from build123d import *

# Parameters (mm, degrees)
F0_W     = 65
F0_H     = 110
F1_DEPTH = 1.6
F2_D     = 3.6


with BuildPart() as f1:
    # F0 (on Top) → F1 (new body)
    with BuildSketch(Plane.XY):
        with Locations((32.5, 55)):
            Rectangle(F0_W, F0_H)
    extrude(amount=F1_DEPTH)

    # F2 (through all)
    with Locations(Plane(origin=(0, 0, 0), x_dir=(1, 0, 0), z_dir=(0, 0, -1))):
        with Locations((3.81, -94.76), (61.19, -94.76), (3.81, -3.81), (61.19, -3.81)):
            Hole(F2_D / 2)


solid = f1.part
For this review, take the finished solid that the model builds, in its own axes (mm). Give positions to 0.01 mm unless a question says otherwise; leave off trailing zeros. Order: outer loops, then holes, each group sorted by start corner. A loop starts at its lowest first (then second) coordinate and runs counter-clockwise, first axis right, second up. Notation, with made-up numbers: M 7,-11 L 16,-11 A9 cw 16,-1 Z; hole C 60.5,-14.5 d2. An arc over 180 degrees is marked long. Answer in a Markdown table with one row per item. Add a question column.
(1) Consider section B-B on x = 61.19. State the section outline as (y, z) points.
(2) Wall thickness on probe 1 along X at (y, z) = (94.76, 0.8); probe 2 along Y at (x, z) = (61.19, 0.75): over which ranges is each line inside the solid? List them lowest first. Write a range as [from, to].
(3) Consider section A-A on y = 94.76. State the section outline as (x, z) points, and give its area (3 significant figures).
(4) Mouldability with a two-part tool opening along Y and no side actions: class faces 1 (the face through (60.359, 5.407, 0.811)), 2 (the face through (32, 56, 1.6)) as +Y half, -Y half, draft (parallel to the pull), parting line (faces both ways), or undercut.
(5) For pin 1 (4 mm diameter, centred on x = 61.19, y = 3.81, fed in from -Z); pin 2 (2 mm diameter, centred on x = 3.81, y = 3.81, fed in from +Z), all flat-tipped, find the tip position at first contact; note any pin that passes through.
Evaluation:
| question | item | result |
|---|---|---|
| 1 | outline | M 0,0 L 2.01,0 L 2.01,1.6 L 0,1.6 Z; M 5.61,0 L 92.96,0 L 92.96,1.6 L 5.61,1.6 Z; M 96.56,0 L 110,0 L 110,1.6 L 96.56,1.6 Z |
| 2 | probe 1 | x = [0, 2.01], [5.61, 59.39], [62.99, 65] |
| 2 | probe 2 | y = [0, 2.01], [5.61, 92.96], [96.56, 110] |
| 3 | outline | M 0,0 L 2.01,0 L 2.01,1.6 L 0,1.6 Z; M 5.61,0 L 59.39,0 L 59.39,1.6 L 5.61,1.6 Z; M 62.99,0 L 65,0 L 65,1.6 L 62.99,1.6 Z |
| 3 | area | 92.5 mm^2 |
| 4 | face 1 | undercut |
| 4 | face 2 | draft |
| 5 | pin 1 | stops at z = 0 |
| 5 | pin 2 | passes through |
